Print and shaded views of the part. All mm, measured from the part's lowest x, y and z. A direction names the side the tool comes from. Round coordinates to 2 decimals unless told otherwise and drop trailing zeros. Write each loop counter-clockwise with the first axis right and the second up, starting at its lowest first coordinate (ties: lowest second). Pieces come first, ordered by that corner, then holes. Notation, with made-up numbers: (24.5, 83) -> (46.5, 83) arc R22 cw to (46.5, 112) -> close; hole circle Ø9 at (-19, 54.5). An arc over 180 degrees is marked (long way). Return JSON: item names as keys, results as strings. Group by question number.
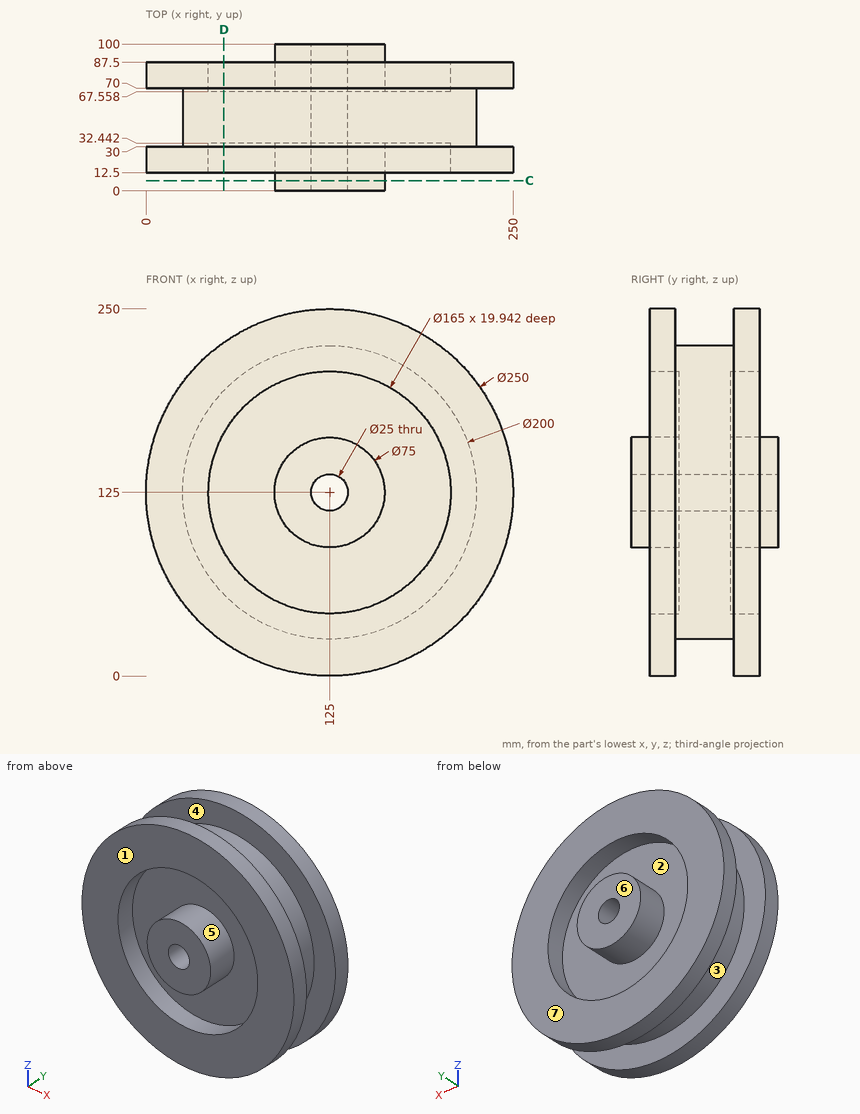
Item 1: Flat gauge pins, fed straight in: P1, Ø12, axis at x = 54, y = 66.5, coming from the -Z side; P2, Ø8, axis at x = 172.5, z = 220.5, coming from the +Y side; P3, Ø3, axis at y = 24.5, z = 138.5, coming from the +X side. Where does each tip first touch, or does it go through?
Item 2: Two-plate mould, pull along Y, no slides. Class the marked faces 1, 2 and 3: released by +Y, released by -Y, zero draft, split by the parting line, or undercut.
Item 3: Which spindle directions (+Z, -Z, +X, -X, +Y, -Y) get a long thin tool onto all of the face, cutting with end or side? Do the marked faces 4, 5, 6 and 7. Say none if no direction does.
Item 4: Cut at D-D (x = 53). Write the cut outline in (y, z), then the cut area to 3 significant figures.
Item 5: Wall check: L1, parallel to X at y = 78.25, z = 125; L2, parallel to Y at x = 57, z = 229.5; L3, parallel to X at y = 45.5, z = 125. Give the ranges that are in metal, low to high.
Item 6: Cut at C-C (y = 7). Write the cut outline in (x, z), then the cut area to 3 significant figures.
Checks:
{
 "1": {"P1": "stops at z = 18.92", "P2": "stops at y = 87.5", "P3": "stops at x = 249.42"},
 "2": {"face 1": "released by -Y", "face 2": "released by +Y", "face 3": "undercut"},
 "3": {"face 4": "none", "face 5": "-Y", "face 6": "+Z, -Z, +X, -X, +Y", "face 7": "+Y"},
 "4": {"outline": "(12.5, 22.82) -> (30, 22.82) -> (30, 55.6) -> (70, 55.6) -> (70, 22.82) -> (87.5, 22.82) -> (87.5, 84.72) -> (67.56, 84.72) -> (67.56, 165.28) -> (87.5, 165.28) -> (87.5, 227.18) -> (70, 227.18) -> (70, 194.4) -> (30, 194.4) -> (30, 227.18) -> (12.5, 227.18) -> (12.5, 165.28) -> (32.44, 165.28) -> (32.44, 84.72) -> (12.5, 84.72) -> close", "area": "9,490 mm2"},
 "5": {"L1": "x = 0 to 42.5, 87.5 to 112.5, 137.5 to 162.5, 207.5 to 250", "L2": "y = 12.5 to 30, 70 to 87.5", "L3": "x = 25 to 112.5, 137.5 to 225"},
 "6": {"outline": "circle Ø75 at (125, 125); hole circle Ø25 at (125, 125)", "area": "3,930 mm2"}
}
